```python
from build123d import *


with BuildPart() as f1:
    # F0 (on Front) → F1 (revolve)
    with BuildSketch(Plane.XZ):
        with BuildLine():
            Line((-37.6, 9.3), (-37.6, 0))
            Line((-37.6, 0), (-25.15, 0))
            ThreePointArc((-25.15, 0), (-24.65, 0.5), (-24.15, 0))
            Line((-24.15, 0), (-14.986, 0))
            Line((-14.986, 0), (-14.986, 39))
            Line((-14.986, 39), (-12.25, 39))
            Line((-12.25, 39), (-12.25, 44))
            Line((-12.25, 44), (0, 44))
            Line((0, 44), (0, 110.4))
            Line((0, 110.4), (-25.4, 110.4))
            Line((-25.4, 110.4), (-25.4, 102.4))
            Line((-25.4, 102.4), (-17.5, 102.4))
            Line((-17.5, 102.4), (-17.5, 97.4))
            Line((-17.5, 97.4), (-25.4, 76.4))
            Line((-25.4, 76.4), (-25.4, 14.3))
            Line((-25.4, 14.3), (-32.6, 14.3))
            Line((-32.6, 14.3), (-37.6, 9.3))
        make_face()
    revolve(axis=Axis((0, 0, 62.623069), (0, 0, 1)))


solid = f1.part
```
Geometry check sheet. Reference: the model listing, model coordinates, mm. A direction names the side the tool comes from. Give positions to 0.01 mm unless a question says otherwise; leave off trailing zeros. Loops run counter-clockwise (first coordinate to the right, second up) from the corner with the lowest first, then second, coordinate; pieces in that order, holes last. Notation, with made-up numbers: (20, 70.25) - (32, 70.25) arc R29 ccw to (32, 105.25) - close; hole circle Ø2 at (-3, 54.25). An arc over 180 degrees is marked (long way). Use CSV: the item, a comma, the result in double quotes. Start each with the question number.
Q1. Access from +Z, -Z, +X, -X, +Y, -Y to the whole of each face (thin tool, end or side, straight path). Record for faces 1 (the face through (8.151, 36.706, 4.585)), 2 (the face through (-8, 25, 0)), 3 (the face through (-19.5, 16.8, 14.3)), 4 (the face through (-6.586, -10.329, 41.535)), 5 (the face through (-18, -5.67, 93.75)).
Q2. Go/stop test with flat-tipped pins: pin 1 Ø6 at (x, y) = (18, 20) entering from -Z; pin 2 Ø1.5 at (x, z) = (12.5, 35.5) entering from +Y; pin 3 Ø6 at (x, y) = (-12.5, 26) entering from +Z; pin 4 Ø2 at (y, z) = (-10.5, 33.5) entering from +X. Record where each tip stops, or that it passes through.
Q3. Release check for a two-part mould opening along X. For faces 6 (the face through (13.887, 10.648, 99.865)), 7 (the face through (1.95, -14.86, 19.77)), 8 (the face through (6, 17, 102.4)) record: +X half, -X half, draft (parallel to the pull), parting line (faces both ways), or undercut.
Q4. Section check C-C, the plane z = 66.5. Record the cut outline in (x, y).
Q5. Scan lines: probe 1 along Y at (x, z) = (0, 42); probe 2 along Y at (x, z) = (0, 17). Record each from-to range of solid material in increasing order. Write a range as from..to.
Findings below:
1,face 1,"+Z, -Z"
1,face 2,"-Z, +X, -X, +Y, -Y"
1,face 3,"+Z"
1,face 4,"-Z"
1,face 5,"none"
2,pin 1,"stops at z = 0"
2,pin 2,"stops at y = 22.52"
2,pin 3,"stops at z = 14.3"
2,pin 4,"stops at x = 23.56"
3,face 6,"parting line"
3,face 7,"undercut"
3,face 8,"draft"
4,outline,"circle Ø50.8 at (0, 0)"
5,probe 1,"y = -25.4..-12.25, 12.25..25.4"
5,probe 2,"y = -25.4..-14.99, 14.99..25.4"
